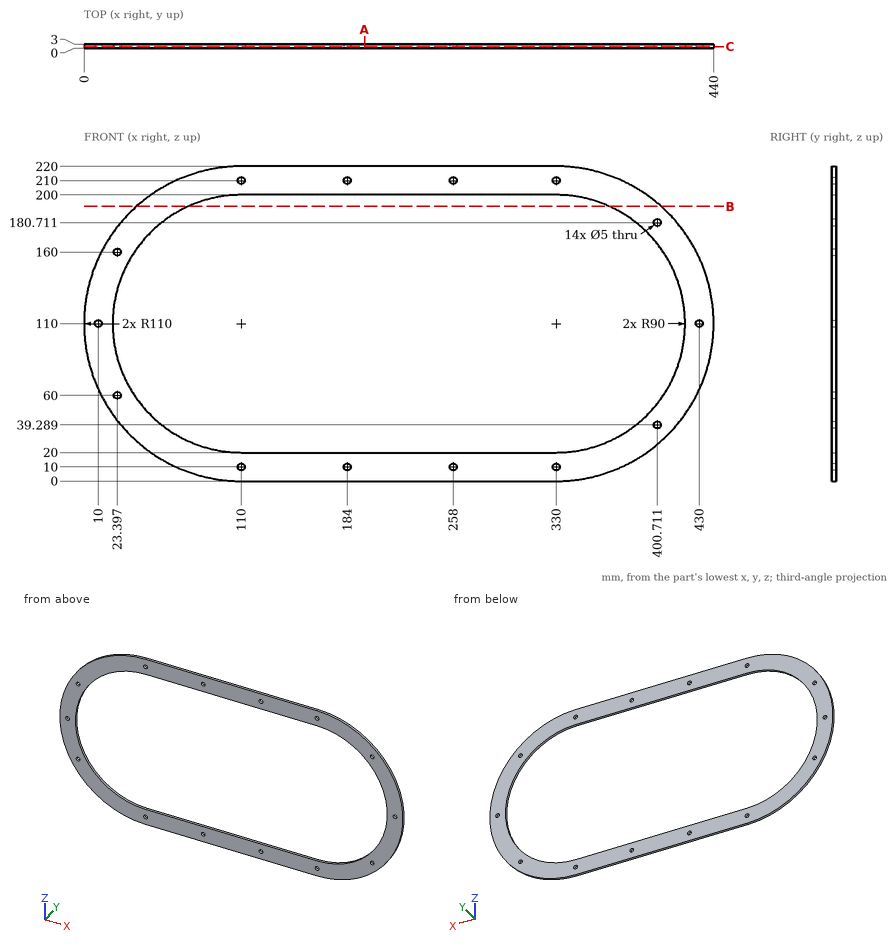
Drawing for the job (mm, zero at the part's lowest x, y, z). Coordinates: 2 decimals unless noted, no trailing zeros. Order: outer loops, then holes, each group sorted by start corner. A loop starts at its lowest first (then second) coordinate and runs counter-clockwise, first axis right, second up. Notation, with made-up numbers: (-16, 68) -> (15, 68) arc R19 cw to (15, 74) -> close; hole circle Ø6 at (-8, 6). An arc over 180 degrees is marked (long way). Return JSON: item names as keys, results as strings.
Item 1: Wall check: line 1 along Z through (x, y) = (330, 0.9); line 2 along X through (y, z) = (1.1, 210) (1 decimal); line 3 along Z through (x, y) = (187.5, 0.55). Give the ranges that are in metal, low to high. Write a range as from..to.
Model answer:
{"line 1": "z = 0..7.5, 12.5..20, 200..207.5, 212.5..220", "line 2": "x = 64.2..107.5, 112.5..181.5, 186.5..255.5, 260.5..327.5, 332.5..375.8", "line 3": "z = 0..20, 200..220"}
Item 2: Pin check, flat tips, straight feed: P1, Ø6.5, axis at x = 110, z = 10, coming from the +Y side; P2, Ø1.5, axis at y = 1.5, z = 74, coming from the +X side. Stop position of each tip, or through.
Model answer:
{"P1": "stops at y = 3", "P2": "stops at x = 434.2"}
Item 3: Slice it at B-B (z = 192). Write the cut outline in (x, y) (1 decimal).
Model answer:
{"outline": "(36.7, 0) -> (72.9, 0) -> (72.9, 3) -> (36.7, 3) -> close; (367.1, 0) -> (403.3, 0) -> (403.3, 3) -> (367.1, 3) -> close"}
Item 4: Slice it at A-A (x = 196). Write the cut outline in (y, z).
Model answer:
{"outline": "(0, 0) -> (3, 0) -> (3, 20) -> (0, 20) -> close; (0, 200) -> (3, 200) -> (3, 220) -> (0, 220) -> close"}
Item 5: Slice it at C-C (y = 1.2). Count the separate pieces of the cut face and the enclosed holes in it, then the cut area to 3 significant figures.
Model answer:
{"separate pieces": "1", "enclosed holes": "15", "area": "21,100 mm²"}
